from build123d import *

# Parameters (mm, degrees)
SKETCH1_W           = 90
SKETCH1_H           = 80
SKETCH1_R           = 2.25
SKETCH1_R_2         = 1.65
SKETCH1_R_3         = 1.25
SKETCH1_W_2         = 32
SKETCH1_H_2         = 62
SKETCH1_W_3         = 25
SKETCH1_H_3         = 45.5
BOSS_EXTRUDE1_DEPTH = 5
CHAMFER1_SIZE       = 15
FILLET1_R           = 3


with BuildPart() as part:
    # Sketch1 → Boss-Extrude1 (new body)
    with BuildSketch(Plane(origin=(0, 0, 0), x_dir=(1, 0, 0), z_dir=(0, 1, 0))):
        Rectangle(SKETCH1_W, SKETCH1_H)
        with Locations(Location((-25, 35, 0), (0, 0, 270))):
            Circle(SKETCH1_R, mode=Mode.SUBTRACT)
        with Locations(Location((25, 35, 0), (0, 0, 90))):
            Circle(SKETCH1_R, mode=Mode.SUBTRACT)
        with Locations(Location((-41.5, 23, 0), (0, 0, 270))):
            Circle(SKETCH1_R_2, mode=Mode.SUBTRACT)
        with Locations(Location((-4.5, 23, 0), (0, 0, 270))):
            Circle(SKETCH1_R_2, mode=Mode.SUBTRACT)
        with Locations(Location((-4.5, -34.5, 0), (0, 0, 270))):
            Circle(SKETCH1_R_2, mode=Mode.SUBTRACT)
        with Locations(Location((-41.5, -34.5, 0), (0, 0, 270))):
            Circle(SKETCH1_R_2, mode=Mode.SUBTRACT)
        with Locations(Location((4, 16, 0), (0, 0, 270))):
            Circle(SKETCH1_R_3, mode=Mode.SUBTRACT)
        with Locations(Location((42, 16, 0), (0, 0, 270))):
            Circle(SKETCH1_R_3, mode=Mode.SUBTRACT)
        with Locations(Location((42, -24, 0), (0, 0, 270))):
            Circle(SKETCH1_R_3, mode=Mode.SUBTRACT)
        with Locations(Location((4, -24, 0), (0, 0, 270))):
            Circle(SKETCH1_R_3, mode=Mode.SUBTRACT)
        with Locations((23, -4)):
            Rectangle(SKETCH1_W_2, SKETCH1_H_2, mode=Mode.SUBTRACT)
        with Locations((-23, -5.75)):
            Rectangle(SKETCH1_W_3, SKETCH1_H_3, mode=Mode.SUBTRACT)
    extrude(amount=BOSS_EXTRUDE1_DEPTH)

    # Chamfer1
    chamfer1_edges = [part.edges().sort_by_distance(p)[0] for p in [
        (-45, 2.5, -40),
        (45, 2.5, -40),
    ]]
    chamfer(chamfer1_edges, length=CHAMFER1_SIZE)

    # Fillet1
    fillet1_edges = [part.edges().sort_by_distance(p)[0] for p in [
        (7, 2.5, -27),
        (7, 2.5, 35),
        (39, 2.5, 35),
        (39, 2.5, -27),
        (-35.5, 2.5, -17),
        (-35.5, 2.5, 28.5),
        (-10.5, 2.5, 28.5),
        (-10.5, 2.5, -17),
        (45, 2.5, 40),
        (-45, 2.5, 40),
        (-30, 2.5, -40),
        (30, 2.5, -40),
        (45, 2.5, -25),
        (-45, 2.5, -25),
    ]]
    fillet(fillet1_edges, radius=FILLET1_R)


solid = part.part
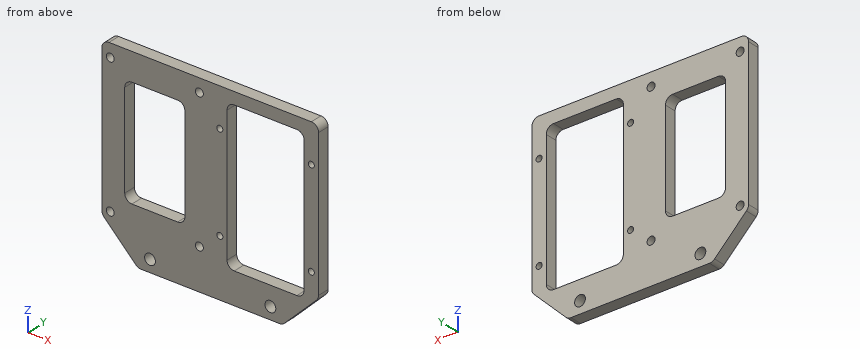
Part model, mm, in its own coordinate system. Coordinates: 2 decimals unless noted, no trailing zeros. Order: outer loops, then holes, each group sorted by start corner. A loop starts at its lowest first (then second) coordinate and runs counter-clockwise, first axis right, second up.
(1) Probe L1, parallel to X at y = 3.85, z = 24; L2, parallel to X at y = 4.3, z = -4; L3, parallel to Z at x = -27, y = 2.95. List the from-to ranges inside material, lowest first.
Check sheet entries:
L1: x = -45 to -35.5, -10.5 to 2.75, 5.25 to 7, 39 to 40.75, 43.25 to 45
L2: x = -45 to -35.5, -10.5 to 7, 39 to 45
L3: z = -40 to -36.03, -33.97 to -17, 28.5 to 40
(2) Slice it at C-C, the plane x = 14. Write the cut outline in (y, z), and give its area (3 significant figures).
Check sheet entries:
outline: (0, -40) - (5, -40) - (5, -27) - (0, -27) - close; (0, 35) - (5, 35) - (5, 40) - (0, 40) - close
area: 90.0 mm2
(3) Slice it at A-A, the plane z = -35. Write the cut outline in (x, y).
Check sheet entries:
outline: (-35, 0) - (-27.25, 0) - (-27.25, 5) - (-35, 5) - close; (-22.75, 0) - (22.75, 0) - (22.75, 5) - (-22.75, 5) - close; (27.25, 0) - (35, 0) - (35, 5) - (27.25, 5) - close
(4) Slice it at B-B, the plane x = 4. Write the cut outline in (y, z), and give its area (3 significant figures).
Check sheet entries:
outline: (0, -40) - (5, -40) - (5, -17.25) - (0, -17.25) - close; (0, -14.75) - (5, -14.75) - (5, 22.75) - (0, 22.75) - close; (0, 25.25) - (5, 25.25) - (5, 40) - (0, 40) - close
area: 375 mm2
(5) Pin check, flat tip, straight feed: pin 1 Ø4 at (x, z) = (42, 24) entering from +Y. Stop position of the tip, or through.
Check sheet entries:
pin 1: stops at y = 5
(6) Slice it at D-D, the plane z = -16. Write the cut outline in (x, y), and give its area (3 significant figures).
Check sheet entries:
outline: (-45, 0) - (-34.74, 0) - (-34.74, 5) - (-45, 5) - close; (-11.26, 0) - (2.75, 0) - (2.75, 5) - (-11.26, 5) - close; (5.25, 0) - (7, 0) - (7, 5) - (5.25, 5) - close; (39, 0) - (40.75, 0) - (40.75, 5) - (39, 5) - close; (43.25, 0) - (45, 0) - (45, 5) - (43.25, 5) - close
area: 148 mm2
